```python
from build123d import *

# Parameters (mm, degrees)
SKETCH1_W                   = 84.137862113
SKETCH1_H                   = 330.949999988
BOSS_EXTRUDE1_DEPTH         = 19.05
HOLE1_D                     = 3.175
HOLE1_DEPTH                 = 31.75
HOLE1_CSINK_D               = 10.16
HOLE1_CSINK_ANGLE           = 82
HOLE1_TIP                   = 0.953866233
HOLE3_D                     = 3.175
HOLE3_DEPTH                 = 38.1
HOLE3_CSINK_D               = 10.16
HOLE3_CSINK_ANGLE           = 82
HOLE3_TIP                   = 0.953866233
F_1_4_0_25_DIAMETER_HOLE1_D = 6.35
HOLE4_D                     = 3.175
HOLE4_DEPTH                 = 31.75
HOLE4_CSINK_D               = 10.16
HOLE4_CSINK_ANGLE           = 82
HOLE4_TIP                   = 0.953866233
HOLE5_D                     = 3.175
HOLE5_DEPTH                 = 38.1
HOLE5_CSINK_D               = 10.16
HOLE5_CSINK_ANGLE           = 82
HOLE5_TIP                   = 0.953866233


with BuildPart() as part:
    # Sketch1 → Boss-Extrude1 (new body)
    with BuildSketch(Plane.XY):
        with Locations((251.421898238, -72.024999997)):
            Rectangle(SKETCH1_W, SKETCH1_H)
    extrude(amount=BOSS_EXTRUDE1_DEPTH)

    # Hole1
    with Locations(Plane(origin=(196.652967181, -72.024999997, 386.262770337), x_dir=(0, 1, 0), z_dir=(-1, 0, 0))):
        with Locations((174.999999994, 685.961004241), (174.999999994, 549.837259632), (174.999999994, 413.713515022), (81.549999997, 779.649723129), (81.549999997, 652.344645962), (62.499999997, 662.953402392), (62.499999997, 769.040966698), (-62.499999997, 769.040966698), (-62.499999997, 662.953402392), (-81.549999997, 652.344645962), (-81.549999997, 779.649723129), (-174.999999994, 413.713515022), (-174.999999994, 549.837259632), (-174.999999994, 685.961004241), (-82.737499997, 600.384620239), (0, 600.384620239), (82.737499997, 600.384620239), (0, 376.737770337), (-82.737499997, 376.737770337), (82.737499997, 376.737770337)):
            CounterSinkHole(HOLE1_D / 2, HOLE1_CSINK_D / 2, depth=HOLE1_DEPTH, counter_sink_angle=HOLE1_CSINK_ANGLE)
            with Locations((0, 0, -(HOLE1_DEPTH + HOLE1_TIP / 2))):  # 118° drill point
                Cone(0, HOLE1_D / 2, HOLE1_TIP, mode=Mode.SUBTRACT)

    # Hole3
    with Locations(Plane(origin=(-181.039434513, 112.499999997, 386.262770337), x_dir=(0.9271838545667855, -1.3196841813264566e-15, -0.37460659341591657), z_dir=(0, 1, 0))):
        with Locations((46.221112845, 113.488854888), (39.39759596, 37.945520226), (412.28786892, 80.423559293), (407.308516105, 25.297013484), (513.561319184, 161.164706775), (597.46020397, 127.267357003), (610.543339245, 159.649253123), (694.322923815, 367.011001477), (526.644454459, 193.546602895), (610.424039029, 400.908351249)):
            CounterSinkHole(HOLE3_D / 2, HOLE3_CSINK_D / 2, depth=HOLE3_DEPTH, counter_sink_angle=HOLE3_CSINK_ANGLE)
            with Locations((0, 0, -(HOLE3_DEPTH + HOLE3_TIP / 2))):  # 118° drill point
                Cone(0, HOLE3_D / 2, HOLE3_TIP, mode=Mode.SUBTRACT)

    # 1/4 (0.25) Diameter Hole1 (through all)
    with Locations(Plane(origin=(0, 0, 0), x_dir=(-1, 0, 0), z_dir=(0, 0, -1))):
        with Locations((-263.328329294, -72.024999997)):
            Hole(F_1_4_0_25_DIAMETER_HOLE1_D / 2)

    # Hole4
    with Locations(Plane(origin=(196.652967181, -72.024999997, 609.90962024), x_dir=(0, 1, 0), z_dir=(-1, 0, 0))):
        with Locations((174.999999994, 685.961004241), (174.999999994, 549.837259632), (174.999999994, 413.713515022), (81.549999997, 779.649723129), (81.549999997, 652.344645962), (62.499999997, 662.953402392), (62.499999997, 769.040966698), (-62.499999997, 769.040966698), (-62.499999997, 662.953402392), (-81.549999997, 652.344645962), (-81.549999997, 779.649723129), (-174.999999994, 413.713515022), (-174.999999994, 549.837259632), (-174.999999994, 685.961004241), (-82.737499997, 600.384620239), (0, 600.384620239), (82.737499997, 600.384620239), (0, 376.737770337), (-82.737499997, 376.737770337), (82.737499997, 376.737770337)):
            CounterSinkHole(HOLE4_D / 2, HOLE4_CSINK_D / 2, depth=HOLE4_DEPTH, counter_sink_angle=HOLE4_CSINK_ANGLE)
            with Locations((0, 0, -(HOLE4_DEPTH + HOLE4_TIP / 2))):  # 118° drill point
                Cone(0, HOLE4_D / 2, HOLE4_TIP, mode=Mode.SUBTRACT)

    # Hole5
    with Locations(Plane(origin=(-181.039434513, 112.499999997, 609.90962024), x_dir=(0.9271838545667913, -6.190403823971236e-15, -0.3746065934159023), z_dir=(0, 1, 0))):
        with Locations((46.221112845, 113.488854888), (39.39759596, 37.945520226), (412.28786892, 80.423559293), (407.308516105, 25.297013484), (513.561319184, 161.164706775), (597.46020397, 127.267357003), (610.413630265, 158.37956732), (694.652415845, 366.877878057), (526.881492954, 193.157790175), (610.762859894, 400.771458735)):
            CounterSinkHole(HOLE5_D / 2, HOLE5_CSINK_D / 2, depth=HOLE5_DEPTH, counter_sink_angle=HOLE5_CSINK_ANGLE)
            with Locations((0, 0, -(HOLE5_DEPTH + HOLE5_TIP / 2))):  # 118° drill point
                Cone(0, HOLE5_D / 2, HOLE5_TIP, mode=Mode.SUBTRACT)


solid = part.part
```
Source: CAD feature listing. Evaluate the final solid. Frame: model axes, mm. Round coordinates to 2 decimals unless told otherwise and drop trailing zeros. Use CSV: the item, a comma, the result in double quotes.
(1) Ray query, L1, parallel to Y at x = 229, z = 9.5; L2, parallel to Y at x = 265, z = 15.25. Return the intervals inside material, ascending.
Report:
L1,"-237.5 to -155.36, -154.17 to -72.62, -71.43 to 10.12, 11.31 to 93.45"
L2,"-237.5 to -74.72, -69.33 to 93.45"
(2) Pull-direction query (Y, two-part tool) for faces 1 (the face through (251, -70, 0)), 2 (the face through (251, 93.45, 9)), 3 (the face through (266.357, -71.071, 9.658)), 4 (the face through (251, -237.5, 9)); classes: +Y half, -Y half, draft (parallel to the pull), parting line (faces both ways), or undercut.
Report:
face 1,"draft"
face 2,"+Y half"
face 3,"undercut"
face 4,"-Y half"
(3) First-contact query: pin 1 Ø8 at (x, y) = (222.5, -172.5) entering from -Z. Flat tip, straight axial feed; report the tip coordinate or a pass-through.
Report:
pin 1,"z = 0"
